Geometry: final body of the model. Coordinates: model frame, mm. A direction names the side the tool comes from. Round coordinates to 2 decimals unless told otherwise and drop trailing zeros. Loops run counter-clockwise (first coordinate to the right, second up) from the corner with the lowest first, then second, coordinate; pieces in that order, holes last. Notation, with made-up numbers: M -34,59.5 L 18,59.5 A25 cw 18,74.5 Z; hole C 69.25,-30 d11. An arc over 180 degrees is marked long. Answer as a JSON object with one key per item and string values.
```python
from build123d import *

# Parameters (mm, degrees)
F1_DEPTH = 15
F2_R     = 4
F3_DEPTH = 20
F4_R     = 5


with BuildPart() as f1:
    # F0 (on Right) → F1 (new body)
    with BuildSketch(Plane.YZ):
        with BuildLine():
            ThreePointArc((-2.222222, -19.87616), (-20, 0), (-2.222222, 19.87616))
            Line((-2.222222, 19.87616), (-91.111111, 9.93808))
            ThreePointArc((-91.111111, 9.93808), (-83.333333, 7.45356), (-80, 0))
            ThreePointArc((-80, 0), (-83.333333, -7.45356), (-91.111111, -9.93808))
            Line((-91.111111, -9.93808), (-2.222222, -19.87616))
        make_face()
        with BuildLine():
            ThreePointArc((-2.222222, -19.87616), (13.333333, -14.90712), (20, 0))
            ThreePointArc((20, 0), (13.333333, 14.90712), (-2.222222, 19.87616))
            ThreePointArc((-2.222222, 19.87616), (-20, 0), (-2.222222, -19.87616))
        make_face()
        with BuildLine():
            ThreePointArc((-80, 0), (-83.333333, 7.45356), (-91.111111, 9.93808))
            ThreePointArc((-91.111111, 9.93808), (-100, 0), (-91.111111, -9.93808))
            ThreePointArc((-91.111111, -9.93808), (-83.333333, -7.45356), (-80, 0))
        make_face()
    extrude(amount=F1_DEPTH)

    # F2 (on Right) → F3 (join)
    with BuildSketch(Plane.YZ):
        with Locations((-90, 0)):
            Circle(F2_R)
    extrude(amount=-F3_DEPTH)

    # F4
    f4_edges = [f1.edges().sort_by_distance(p)[0] for p in [
        (15, 13.333333, -14.90712),
        (15, 13.333333, 14.90712),
        (15, -46.666667, 14.90712),
        (15, -100, 0),
        (15, -46.666667, -14.90712),
    ]]
    fillet(f4_edges, radius=F4_R)


solid = f1.part
```
1) Line query: probe 1 along X at (y, z) = (-6.5, 3); probe 2 along X at (y, z) = (14, -12); probe 3 along Y at (x, z) = (10, 8). Output: solid intervals per line, ascending.
Geometry results:
{"probe 1": "0 to 15", "probe 2": "0 to 13.63", "probe 3": "-96 to 18.33"}
2) Set-up query: faces 1 (the face through (-10, -94, 0)), 2 (the face through (13.574, -47.122, 13.343)). Return all of +Z, -Z, +X, -X, +Y, -Y with unobstructed straight access to the full face (end or side cutting, diameter ignored); none if empty.
Geometry results:
{"face 1": "-X", "face 2": "+Z, +X, -Y"}
3) Cut plane A-A on x = 6. Return the cut outline in (y, z), and give its area (3 significant figures).
Geometry results:
{"outline": "M -91.11,-9.94 L -2.22,-19.88 A20 ccw long -2.22,19.88 L -91.11,9.94 A10 ccw Z", "area": "3,500 mm2"}
4) First-contact query: pin 1 (10 mm diameter, centred on x = -8.5, z = 1.5, fed in from -Y); pin 2 (20 mm diameter, centred on y = -58, z = -8.5, fed in from -X); pin 3 (6 mm diameter, centred on x = 0, z = -6.5, fed in from -Y). Flat tips, straight axial feed; report the tip coordinate or a pass-through.
Geometry results:
{"pin 1": "y = -94", "pin 2": "x = 0", "pin 3": "y = -99.37"}
5) Cut plane B-B on x = -4.5. Return the cut outline in (y, z).
Geometry results:
{"outline": "C -90,0 d8"}
